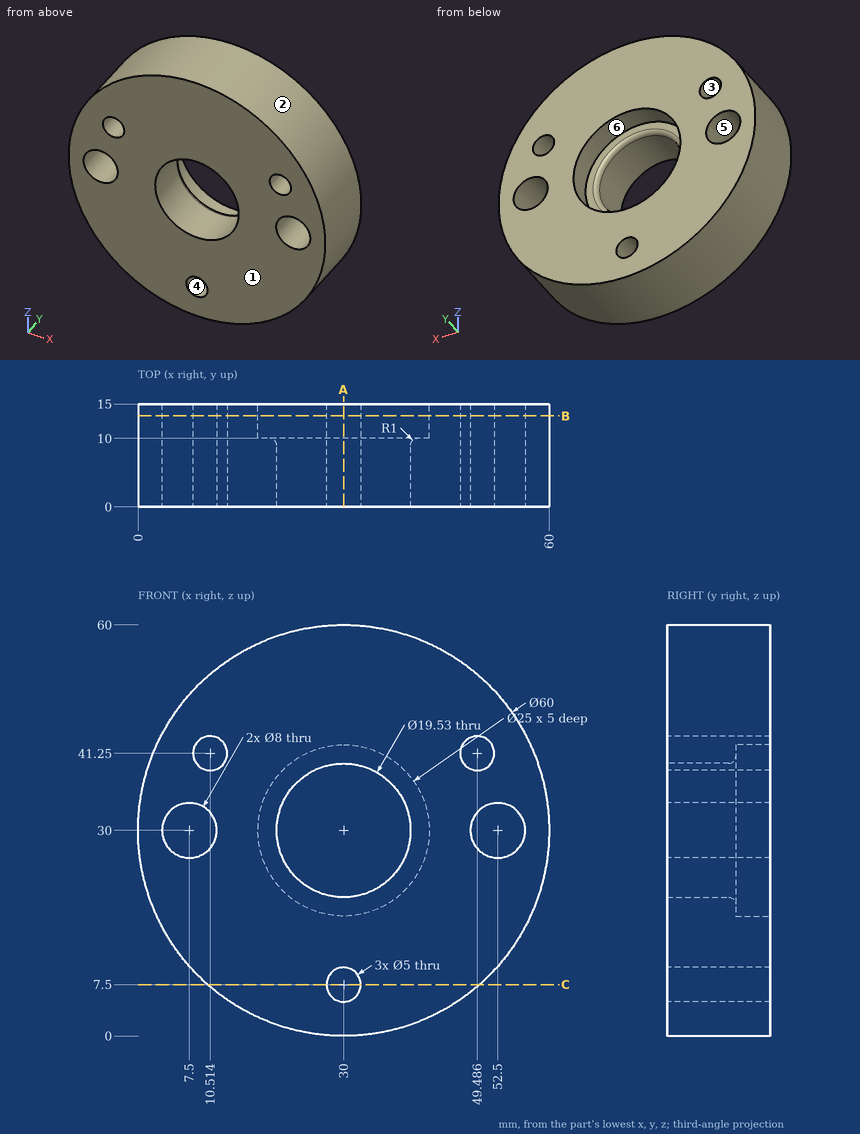
Part print with two shaded views. Sizes in mm from the minimum x, y, z corner. A direction names the side the tool comes from. Round coordinates to 2 decimals unless told otherwise and drop trailing zeros. Order: outer loops, then holes, each group sorted by start corner. A loop starts at its lowest first (then second) coordinate and runs counter-clockwise, first axis right, second up.
(1) Band-saw the part on A-A (x = 30). List the corners of the cut face in (y, z) (1 decimal), then the cut area to 3 significant figures.
(2) 3-axis set-ups, long thin cutter, end or side, ignore diameter. For the marked faces 5 and 6: which of +Z, -Z, +X, -X, +Y, -Y reach the whole face in a straight line?
(3) Band-saw the part on C-C (z = 7.5). List the corners of the cut face in (x, y), then the cut area to 3 significant figures.
(4) Pull direction Z, two halves, no side cores. Call the marked faces 1, 2, 3 and 4: released by +Z, released by -Z, zero draft, split by the parting line, or undercut.
(5) Pin check, flat tips, straight feed: pin 1 (12.5 mm diameter, centred on x = 25.5, z = 31.5, fed in from +Y); pin 2 (4.5 mm diameter, centred on x = 10.51, z = 41.25, fed in from +Y); pin 3 (5 mm diameter, centred on x = 49, y = 2.5, fed in from -Z) (1 decimal); pin 4 (5 mm diameter, centred on y = 11, z = 26.5, fed in from -X). Stop position of each tip, or through.
(6) Drill centre lines: line 1 (X direction, y = 13.05, z = 30); line 2 (X direction, y = 6.75, z = 30) (1 decimal); line 3 (X direction, y = 6.5, z = 41.25) (1 decimal). Where is each one in solid material? Low to high.
(7) Band-saw the part on B-B (y = 13.25). Give the number of separate pieces and of enclosed holes in the cut face, then the cut area to 3 significant figures.
Verdict:
1. outline: (0, 0) - (15, 0) - (15, 5) - (0, 5) - close; (0, 10) - (15, 10) - (15, 17.5) - (10, 17.5) - (10, 19.2) arc R1 ccw to (9, 20.2) - (0, 20.2) - close; (0, 39.8) - (9, 39.8) arc R1 ccw to (10, 40.8) - (10, 42.5) - (15, 42.5) - (15, 60) - (0, 60) - close
1. area: 504 mm2
2. face 5: +Y, -Y
2. face 6: +Y
3. outline: (10.16, 0) - (27.5, 0) - (27.5, 15) - (10.16, 15) - close; (32.5, 0) - (49.84, 0) - (49.84, 15) - (32.5, 15) - close
3. area: 520 mm2
4. face 1: zero draft
4. face 2: split by the parting line
4. face 3: undercut
4. face 4: undercut
5. pin 1: stops at y = 10
5. pin 2: passes through
5. pin 3: stops at z = 4.9
5. pin 4: stops at x = 0.02
6. line 1: x = 0 to 3.5, 11.5 to 17.5, 42.5 to 48.5, 56.5 to 60
6. line 2: x = 0 to 3.5, 11.5 to 20.2, 39.8 to 48.5, 56.5 to 60
6. line 3: x = 2.2 to 8, 13 to 47, 52 to 57.8
7. separate pieces: 1
7. enclosed holes: 6
7. area: 2,180 mm2
